Can you work these out from the model? Positions are in its coordinate system, mm. A direction names the side the tool comes from. Coordinates: 2 decimals unless noted, no trailing zeros. Order: outer loops, then holes, each group sorted by start corner. A loop starts at its lowest first (then second) coordinate and runs counter-clockwise, first axis right, second up. Notation, with made-up numbers: (24.25, -34) -> (63.25, -34) arc R19 cw to (63.25, -26) -> close; hole circle Ø11 at (-1, 83). An arc over 180 degrees is marked (long way). Answer as a JSON object with one key per item and string values. Group by question number.
(1) Which directions (+Z, -Z, +X, -X, +Y, -Y) give clear straight access to the entire face, cutting with the end or side of a thin tool? Please do faces 4 (the cylindrical face through (-0.207, 6.261, 14.274)), 5 (the cylindrical face through (-3.441, 7.871, -15.497)).
(2) I want a section at B-B, the plane z = 10. List the corners of the cut face in (x, y) for me (3 decimals).
(3) I want a section at A-A, the plane x = 0. State how many separate pieces and enclosed holes the cut face has, plus the area to 3 significant figures.
(4) I want a section at D-D, the plane x = -5.5. List the corners of the cut face in (y, z) for me (3 decimals).
(5) I want a section at C-C, the plane x = 12.7. List the corners of the cut face in (y, z) for me (1 decimal).
(6) I need wall thicknesses on line 1 (Z direction, x = 0, y = 8) (1 decimal); line 2 (Z direction, x = 1, y = 5); line 3 (Z direction, x = -4.5, y = 9.5). Which ranges of each line are inside material? Lowest first, please.
(7) If we mould it in two halves opening along Z, with no side actions, what happens to faces 1 (the cylindrical face through (15.12, 1.57, 11.59)), 2 (the flat face through (4, 3.175, 16)), 3 (the cylindrical face through (-2.976, 6.261, 4.967))? For each: pulls with the +Z half, pulls with the -Z half, needs draft (parallel to the pull), parting line crosses it, or undercut.
(8) For pin 1 (3 mm diameter, centred on x = -4.49, z = 4.49, fed in from -Y); pin 2 (5 mm diameter, centred on y = 7, z = -8.5, fed in from -X); pin 3 (5 mm diameter, centred on x = -9, y = 7, fed in from -Z); pin 4 (4 mm diameter, centred on y = 3, z = 12, fed in from -X), each with a flat end and sliding along its axis, tell me the tip position at first contact or that it passes through.
Autodesk Inventor part; units mm, degrees
ref_plane "YZ Plane" through (0, 0, 0) normal (1, 0, 0) x (0, 1, 0)
ref_plane "XZ Plane" through (0, 0, 0) normal (0, 1, 0) x (-1, 0, 0)
ref_plane "XY Plane" through (0, 0, 0) normal (0, 0, 1) x (1, 0, 0)
sketch "Sketch1" plane through (0, 0, 0) normal (0, 1, 0) x (-1, 0, 0)
  circle A0 centre (0, 0) radius 19.05
  circle A1 centre (0, 0) radius 12.7
  dimension "d0" = 38.1
  dimension "d1" = 25.4
extrude "Extrusion1" add sketch "Sketch1" along normal blind 3.175
sketch "Sketch2" plane through (0, 3.175, 0) normal (0, 1, 0) x (1, 0, 0)
  circle A0 centre (0, 0) radius 12.7
  circle A1 centre (0, 0) radius 19.05
  circle A2 centre (0, 0) radius 15.875
  dimension "d4" = 31.75
extrude "Extrusion2" add sketch "Sketch2" along normal blind 9.525 contours A2
sketch "Sketch4" plane through (0, 12.7, 0) normal (0, 1, 0) x (1, 0, 0)
  circle A0 centre (0, 0) radius 12.7
  circle A1 centre (0, 0) radius 15.875
extrude "Extrusion4" add sketch "Sketch4" against normal up to surface (12.7 mm away) contours A0
sketch "Sketch5" plane through (0, 0, 0) normal (0, -1, 0) x (1, 0, 0)
  circle A0 centre (-6.35, 0) radius 1.5875
  circle A1 centre (-12.7, 0) radius 1.5875
  circle A2 centre (0, -6.35) radius 1.5875
  circle A3 centre (0, -12.7) radius 1.5875
  circle A4 centre (6.35, 0) radius 1.5875
  circle A5 centre (12.7, 0) radius 1.5875
  circle A6 centre (4.4901, 4.4901) radius 1.5875
  circle A7 centre (8.9803, 8.9803) radius 1.5875
  circle A8 centre (8.9803, -8.9803) radius 1.5875
  circle A9 centre (4.4901, -4.4901) radius 1.5875
  circle A10 centre (-8.9803, -8.9803) radius 1.5875
  circle A11 centre (-4.4901, -4.4901) radius 1.5875
  circle A12 centre (-8.9803, 8.9803) radius 1.5875
  circle A13 centre (-4.4901, 4.4901) radius 1.5875
  circle A14 centre (0, 6.35) radius 1.5875
  circle A15 centre (0, 12.7) radius 1.5875
  circle A16 centre (0, 0) radius 1.5875
  circle A17 centre (0, 0) radius 15.875
extrude "Extrusion5" cut sketch "Sketch5" against normal through all contours A0 | A1 | A2 | A3 | A4 | A5 | A6 | A7 | A8 | A9 | A10 | A11 | A12 | A13 | A14 | A15 | A16
properties part number "insideFlange" material "Polycarbonate, Clear"
Computed values:
{
 "1": {"face 4": "+Y, -Y", "face 5": "+Y"},
 "2": {"outline": "(-16.214, 0) -> (-10.197, 0) -> (-10.197, 12.7) -> (-12.329, 12.7) -> (-12.329, 3.175) -> (-16.214, 3.175) -> close; (-7.764, 0) -> (7.764, 0) -> (7.764, 12.7) -> (-7.764, 12.7) -> close; (10.197, 0) -> (16.214, 0) -> (16.214, 3.175) -> (12.329, 3.175) -> (12.329, 12.7) -> (10.197, 12.7) -> close"},
 "3": {"separate pieces": "6", "enclosed holes": "0", "area": "222 mm2"},
 "4": {"outline": "(0, -18.239) -> (3.175, -18.239) -> (3.175, -14.892) -> (12.7, -14.892) -> (12.7, -5.715) -> (0, -5.715) -> close; (0, -3.265) -> (12.7, -3.265) -> (12.7, -1.341) -> (0, -1.341) -> close; (0, 1.341) -> (12.7, 1.341) -> (12.7, 3.265) -> (0, 3.265) -> close; (0, 5.715) -> (12.7, 5.715) -> (12.7, 14.892) -> (3.175, 14.892) -> (3.175, 18.239) -> (0, 18.239) -> close"},
 "5": {"outline": "(0, -14.2) -> (3.2, -14.2) -> (3.2, -9.5) -> (12.7, -9.5) -> (12.7, -1.6) -> (0, -1.6) -> close; (0, 1.6) -> (12.7, 1.6) -> (12.7, 9.5) -> (3.2, 9.5) -> (3.2, 14.2) -> (0, 14.2) -> close"},
 "6": {"line 1": "z = -15.9 to -14.3, -11.1 to -7.9, -4.8 to -1.6, 1.6 to 4.8, 7.9 to 11.1, 14.3 to 15.9", "line 2": "z = -15.84 to -13.93, -11.47 to -7.58, -5.12 to -1.23, 1.23 to 5.12, 7.58 to 11.47, 13.93 to 15.84", "line 3": "z = -15.22 to -6.08, -2.9 to 2.9, 6.08 to 15.22"},
 "7": {"face 1": "parting line crosses it", "face 2": "needs draft", "face 3": "undercut"},
 "8": {"pin 1": "passes through", "pin 2": "stops at x = -14.7", "pin 3": "stops at z = -14.48", "pin 4": "stops at x = -16.21"}
}
